```python
from build123d import *

# Parameters (mm, degrees)
SKETCH_1_W          = 40
SKETCH_1_H          = 40
EXTRUDE_1_DEPTH     = 50
SKETCH_2_W          = 36
SKETCH_2_H          = 36
CUT_EXTRUDE_1_DEPTH = 46
SKETCH_3_R          = 1.5
CUT_EXTRUDE_2_DEPTH = 46
SKETCH_4_R          = 1.5
CUT_EXTRUDE_3_DEPTH = 46


with BuildPart() as part:
    # 草图1 → 凸台-拉伸1 (new body)
    with BuildSketch(Plane(origin=(0, 0, 0), x_dir=(1, 0, 0), z_dir=(0, 1, 0))):
        with Locations((20, -20)):
            Rectangle(SKETCH_1_W, SKETCH_1_H)
    extrude(amount=EXTRUDE_1_DEPTH)

    # 草图2 → 切除-拉伸1 (cut)
    with BuildSketch(Plane(origin=(0, 50, 0), x_dir=(1, 0, 0), z_dir=(0, 1, 0))):
        with Locations((20, -20)):
            Rectangle(SKETCH_2_W, SKETCH_2_H)
    extrude(amount=-CUT_EXTRUDE_1_DEPTH, mode=Mode.SUBTRACT)

    # 草图3 → 切除-拉伸2 (cut)
    with BuildSketch(Plane.XY.offset(40)):
        with Locations((20, 38)):
            Circle(SKETCH_3_R)
    extrude(amount=-CUT_EXTRUDE_2_DEPTH, mode=Mode.SUBTRACT)

    # 草图4 → 切除-拉伸3 (cut)
    with BuildSketch(Plane(origin=(40, 0, 0), x_dir=(0, 0, -1), z_dir=(1, 0, 0))):
        with Locations((-20, 38)):
            Circle(SKETCH_4_R)
    extrude(amount=-CUT_EXTRUDE_3_DEPTH, mode=Mode.SUBTRACT)


solid = part.part
```
Build history of the part. All positions in model axes, mm. A direction names the side the tool comes from. Round coordinates to 2 decimals unless told otherwise and drop trailing zeros. Loops run counter-clockwise (first coordinate to the right, second up) from the corner with the lowest first, then second, coordinate; pieces in that order, holes last.
Item 1: Saw through at A-A (z = 20). List the corners of the cut face in (x, y).
Item 2: Saw through at D-D (x = 11.5). List the corners of the cut face in (y, z), then the cut area to 3 significant figures.
Item 3: Saw through at C-C (x = 20). List the corners of the cut face in (y, z), then the cut area to 3 significant figures.
Item 4: Saw through at B-B (y = 21). List the corners of the cut face in (x, z), then the cut area to 3 significant figures.
Item 5: Drill centre lines: line 1 along X through (y, z) = (16.5, 22.5); line 2 along Y through (x, z) = (38.65, 20). Where is each one in solid material? Low to high.
Item 6: Two-plate mould, pull along Z, no slides. Class faces 1 (the face through (20, 25, 40)), 2 (the face through (20, 25, 0)), 3 (the face through (39, 37.1, 21.2)): released by +Z, released by -Z, zero draft, split by the parting line, or undercut.
Item 7: Pin check, flat tips, straight feed: P1, Ø1.5, axis at x = 25.5, z = 21.5, coming from the +Y side; P2, Ø6, axis at y = 22, z = 6, coming from the -X side; P3, Ø1.8, axis at y = 38, z = 20, coming from the +X side. Stop position of each tip, or through.
Item 8: Which spindle directions (+Z, -Z, +X, -X, +Y, -Y) get a long thin tool onto all of the face, cutting with end or side? Do faces 4 (the face through (38, 27, 20)), 5 (the face through (18.8, 37.1, 39)). Say none if no direction does.
Worked answers:
1. outline: (0, 0) - (40, 0) - (40, 36.5) - (38, 36.5) - (38, 4) - (2, 4) - (2, 36.5) - (0, 36.5) - close; (0, 39.5) - (2, 39.5) - (2, 50) - (0, 50) - close; (38, 39.5) - (40, 39.5) - (40, 50) - (38, 50) - close
2. outline: (0, 0) - (50, 0) - (50, 2) - (4, 2) - (4, 38) - (50, 38) - (50, 40) - (0, 40) - close
2. area: 344 mm2
3. outline: (0, 0) - (36.5, 0) - (36.5, 2) - (4, 2) - (4, 38) - (36.5, 38) - (36.5, 40) - (0, 40) - close; (39.5, 0) - (50, 0) - (50, 2) - (39.5, 2) - close; (39.5, 38) - (50, 38) - (50, 40) - (39.5, 40) - close
3. area: 332 mm2
4. outline: (0, 0) - (40, 0) - (40, 40) - (0, 40) - close; hole (2, 2) - (38, 2) - (38, 38) - (2, 38) - close
4. area: 304 mm2
5. line 1: x = 0 to 2, 38 to 40
5. line 2: y = 0 to 36.5, 39.5 to 50
6. face 1: released by +Z
6. face 2: released by -Z
6. face 3: undercut
7. P1: stops at y = 4
7. P2: stops at x = 0
7. P3: passes through
8. face 4: +Y
8. face 5: +Z, -Z
